Work out the finished part from the listing and answer in its coordinate system (mm). Face numbers are marked on the shaded views. A direction names the side the tool comes from. Round coordinates to 2 decimals unless told otherwise and drop trailing zeros. Loops run counter-clockwise (first coordinate to the right, second up) from the corner with the lowest first, then second, coordinate; pieces in that order, holes last. Notation, with made-up numbers: (-8, 7.25) - (46, 7.25) arc R16 cw to (46, 38.25) - close; hole circle Ø5 at (27, 88). An arc over 180 degrees is marked (long way). Return JSON: item names as keys, results as strings.
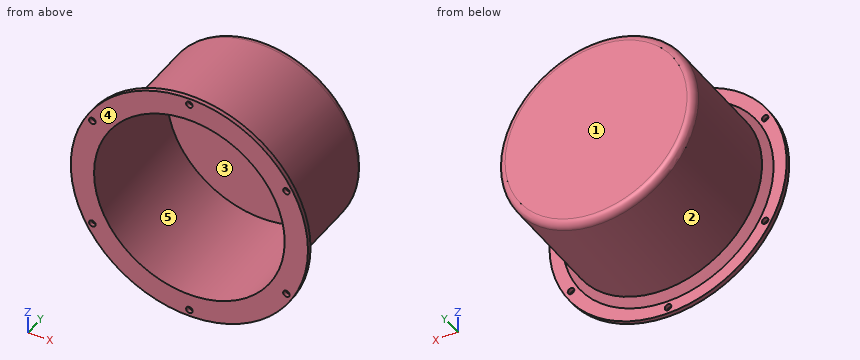
Autodesk Inventor part; units mm, degrees
ref_plane "YZ Plane" through (0, 0, 0) normal (1, 0, 0) x (0, 1, 0)
ref_plane "XZ Plane" through (0, 0, 0) normal (0, 1, 0) x (-1, 0, 0)
ref_plane "XY Plane" through (0, 0, 0) normal (0, 0, 1) x (1, 0, 0)
sketch "Sketch1" plane through (0, 0, 0) normal (0, 0, 1) x (1, 0, 0)
  line L0 (-16.3, 0) -> (97.8, 0) construction
  line L1 (0, 60.9) -> (0, -60.9) construction
  line L2 (65.5, -43.5) -> (65.5, 41.5)
  line L3 (81.5, -40.5) -> (81.5, -43.5)
  line L4 (81.5, -43.5) -> (65.5, -43.5)
  line L5 (67.5, -35.5) -> (67.5, 43.5)
  line L6 (81.5, -40.5) -> (72.5, -40.5)
  line L7 (72.5, -40.5) -> (67.5, -35.5)
  line L8 (67.5, 43.5) -> (0, 43.5)
  line L9 (65.5, 41.5) -> (0, 41.5)
  line L10 (0, 43.5) -> (0, 41.5)
  point P0 (0, 0)
  dimension "d5" = 81.5
  dimension "d7" = 9
  dimension "d8" = 5
  dimension "d9" = 45
  dimension "d10" = 16
  dimension "d11" = 3
  dimension "d30" = 2
  dimension "d32" = 2
  dimension "d34" = 87
revolve "Revolution1" add sketch "Sketch1" angle 360 about axis through (0, 0, 0) along (0, -1, 0)
sketch "Sketch2" plane through (0, -43.5, 0) normal (0, -1, 0) x (1, 0, 0)
  line L0 (0, 114.1) -> (0, -114.1) construction
  line L1 (-114.1, 0) -> (114.1, 0) construction
  circle A0 centre (0, 0) radius 81.5 construction
  circle A1 centre (0, 0) radius 65.5 construction
  circle A2 centre (0, 0) radius 77 construction
  circle A3 centre (0, 0) radius 72.5 construction
  point P0 (0, 77)
  point P1 (-66.684, 38.5)
  point P2 (-66.684, -38.5)
  point P3 (0, -77)
  point P4 (66.684, -38.5)
  point P5 (66.684, 38.5)
  dimension "d16" = 4.5
  dimension "d20" = 360
  dimension "d29" = 4.5
hole "Hole1" at (0, -43.5, 77) at (-66.684, -43.5, 38.5) at (-66.684, -43.5, -38.5) at (0, -43.5, -77) at (66.684, -43.5, -38.5) at (66.684, -43.5, 38.5) direction (0, 1, 0) diameter 4.5 depth 13 tip angle 118
fillet "Fillet1" radius 5 1 edges at (-67.5, 43.5, 0)
equation "\"d16\" = d29"
properties part number "Cover_Joint_1_2" material "Aluminum 6061"
1) Section D-D (y = -2.5) is taken. Give the vertices of the cut face in (x, z), and give its area (3 significant figures).
Verdict:
{"outline": "circle Ø135 at (0, 0); hole circle Ø131 at (0, 0)", "area": "836 mm2"}
2) Section A-A (x = 0) is taken. Give the vertices of the cut face in (y, z).
Verdict:
{"outline": "(-43.5, -81.5) - (-40.5, -81.5) - (-40.5, -79.25) - (-43.5, -79.25) - close; (-43.5, -74.75) - (-40.5, -74.75) - (-40.5, -72.5) - (-35.5, -67.5) - (38.5, -67.5) arc R5 ccw to (43.5, -62.5) - (43.5, 62.5) arc R5 ccw to (38.5, 67.5) - (-35.5, 67.5) - (-40.5, 72.5) - (-40.5, 74.75) - (-43.5, 74.75) - (-43.5, 65.5) - (41.5, 65.5) - (41.5, -65.5) - (-43.5, -65.5) - close; (-43.5, 79.25) - (-40.5, 79.25) - (-40.5, 81.5) - (-43.5, 81.5) - close"}
3) Section C-C (z = -77) is taken. Give the vertices of the cut face in (x, y), and give its area (3 significant figures).
Verdict:
{"outline": "(-26.71, -43.5) - (-2.25, -43.5) - (-2.25, -40.5) - (-26.71, -40.5) - close; (2.25, -43.5) - (26.71, -43.5) - (26.71, -40.5) - (2.25, -40.5) - close", "area": "147 mm2"}
4) Flat-ended cylindrical pins translate along their axes: pin 1 (2 mm diameter, centred on x = 29.5, y = 5, fed in from +Z); pin 2 (5 mm diameter, centred on x = -16.5, z = -64, fed in from +Y); pin 3 (2 mm diameter, centred on y = 11, z = -50.5, fed in from +X); pin 4 (7 mm diameter, centred on x = 66.684, z = -38.5, fed in from -Y). Find the tip coordinate at first contact, or state that the pin passes through.
Verdict:
{"pin 1": "stops at z = 61.19", "pin 2": "stops at y = 43.38", "pin 3": "stops at x = 45.89", "pin 4": "stops at y = -43.5"}
5) Determine the mould class of the marked faces 1, 2 and 3 for opening direction X: pulls with the +X half, pulls with the -X half, needs draft (parallel to the pull), parting line crosses it, or undercut.
Verdict:
{"face 1": "needs draft", "face 2": "parting line crosses it", "face 3": "undercut"}
6) Section B-B (z = 0) is taken. Give the vertices of the cut face in (x, y).
Verdict:
{"outline": "(-81.5, -43.5) - (-65.5, -43.5) - (-65.5, 41.5) - (65.5, 41.5) - (65.5, -43.5) - (81.5, -43.5) - (81.5, -40.5) - (72.5, -40.5) - (67.5, -35.5) - (67.5, 38.5) arc R5 ccw to (62.5, 43.5) - (-62.5, 43.5) arc R5 ccw to (-67.5, 38.5) - (-67.5, -35.5) - (-72.5, -40.5) - (-81.5, -40.5) - close"}
7) A tool of negligible diameter and unlimited length cuts with its end or side. For the marked faces 4 and 5, from which of +Z, -Z, +X, -X, +Y, -Y can it reach the whole face along a straight path? Write none if from no direction.
Verdict:
{"face 4": "+Z, -Z, +X, -X, -Y", "face 5": "-Y"}
8) Find the intervals of material crossed by L1, parallel to X at y = -8, z = -1; L2, parallel to X at y = -41, z = 38; L3, parallel to Z at x = -1.5, y = -27.5, in increasing order.
Verdict:
{"L1": "x = -67.49 to -65.49, 65.49 to 67.49", "L2": "x = -72.1 to -68.88, -64.49 to -53.35, 53.35 to 64.49, 68.88 to 72.1", "L3": "z = -67.48 to -65.48, 65.48 to 67.48"}
